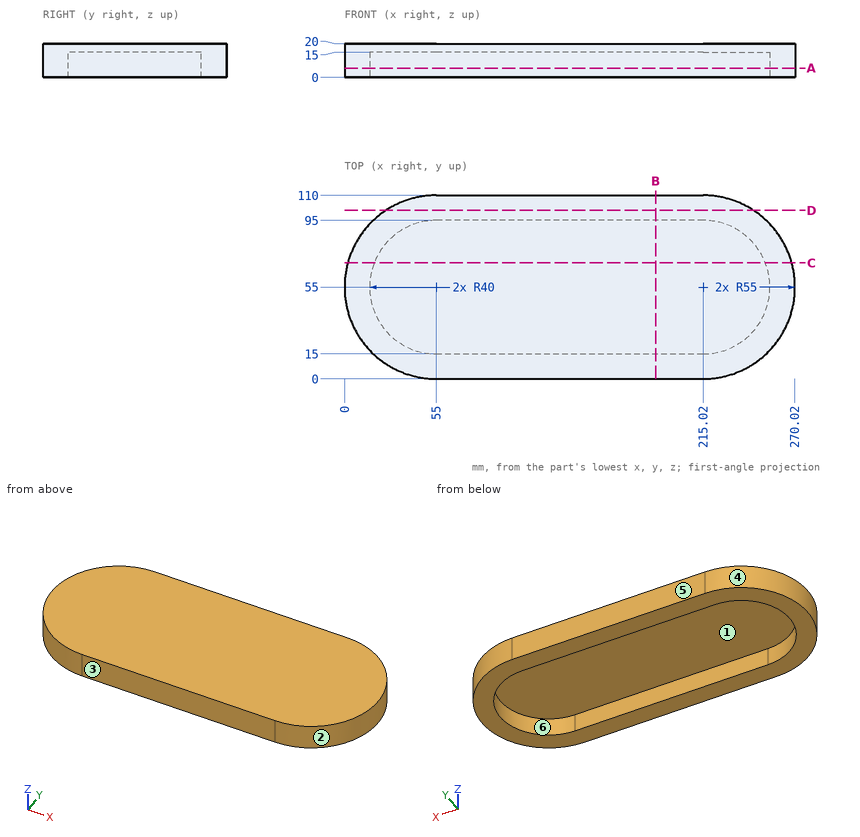
Print and shaded views of the part. All mm, measured from the part's lowest x, y and z. A direction names the side the tool comes from. Coordinates: 2 decimals unless noted, no trailing zeros. Loops run counter-clockwise (first coordinate to the right, second up) from the corner with the lowest first, then second, coordinate; pieces in that order, holes last. Notation, with made-up numbers: (3, 47.5) - (26, 47.5) arc R24 ccw to (26, 74.5) - close; hole circle Ø2 at (-31, 22.5). An arc over 180 degrees is marked (long way). Write item = value, one per line. Start each with the question number.
Item 1: Drop flat-ended pins along their axis: pin 1 Ø5 at (x, y) = (75.5, 69.5) entering from -Z; pin 2 Ø5 at (y, z) = (26, 16) entering from -X (1 decimal); pin 3 Ø1 at (y, z) = (62.5, 5.5) entering from +X. Give the stop position or say it passes through.
Item 2: 3-axis set-ups, long thin cutter, end or side, ignore diameter. For the marked faces 1 and 2: which of +Z, -Z, +X, -X, +Y, -Y reach the whole face in a straight line?
Item 3: Wall check: probe 1 along Y at (x, z) = (211, 8.5); probe 2 along Z at (x, y) = (224, 33); probe 3 along X at (y, z) = (39.5, 10.75) (1 decimal). Give the ranges that are in metal, low to high. Write a range as [from, to].
Item 4: Saw through at C-C, the plane y = 69.5. List the corners of the cut face in (x, z) (1 decimal).
Item 5: Saw through at B-B, the plane x = 186.5. List the corners of the cut face in (y, z), then the cut area to 3 significant figures.
Item 6: Saw through at D-D, the plane y = 101. List the corners of the cut face in (x, z).
Item 7: Saw through at A-A, the plane z = 5.5. List the corners of the cut face in (x, y) (1 decimal).
Item 8: Pull direction Y, two halves, no side cores. Call the marked faces 3, 4, 5 and 6: +Y half, -Y half, draft (parallel to the pull), parting line (faces both ways), or undercut.
Answers:
q1.pin_1 = 15
q1.pin_2 = 6.8
q1.pin_3 = 269.57
q2.face_1 = -Z
q2.face_2 = +Z, -Z, +X
q3.probe_1 = [0, 15], [95, 110]
q3.probe_2 = [15, 20]
q3.probe_3 = [2.2, 18.1], [251.9, 267.8]
q4.outline = (1.9, 0) - (17.7, 0) - (17.7, 15) - (252.3, 15) - (252.3, 0) - (268.1, 0) - (268.1, 20) - (1.9, 20) - close
q5.outline = (0, 0) - (15, 0) - (15, 15) - (95, 15) - (95, 0) - (110, 0) - (110, 20) - (0, 20) - close
q5.area = 1,000 mm2
q6.outline = (24.85, 0) - (245.17, 0) - (245.17, 20) - (24.85, 20) - close
q7.outline = (55, 0) - (215, 0) arc R55 ccw to (215, 110) - (55, 110) arc R55 ccw to start; hole (55, 15) - (215, 15) arc R40 ccw to (215, 95) - (55, 95) arc R40 ccw to start
q8.face_3 = -Y half
q8.face_4 = parting line
q8.face_5 = +Y half
q8.face_6 = undercut
